Model file for the job. Use its own axes, mm. Give positions to 0.01 mm unless a question says otherwise; leave off trailing zeros. Loops run counter-clockwise (first coordinate to the right, second up) from the corner with the lowest first, then second, coordinate; pieces in that order, holes last. Notation, with made-up numbers: M -15.5,52 L -9.5,52 A31 ccw -9.5,77 Z; hole C 63,83 d5. An arc over 180 degrees is marked long. Answer in a Markdown table with one row per item.
```python
from build123d import *

# Parameters (mm, degrees)
F2_R = 10
F3_R = 2


with BuildPart() as f1:
    # F0 (on Front) → F1 (revolve)
    with BuildSketch(Plane.XZ):
        with BuildLine():
            Line((0, 70), (0, 0))
            Line((0, 0), (25.5, 0))
            Line((25.5, 0), (25.5, 12))
            Line((25.5, 12), (23.161351406, 9.536806494))
            Line((23.161351406, 9.536806494), (12.4268941581, 9.536806494))
            Line((12.4268941581, 9.536806494), (8.2896918707, 17.4999870426))
            Line((8.2896918707, 17.4999870426), (17.8353563403, 54.2824750416))
            add(Edge.make_bspline(
                [(17.8353563403, 54.2824750416), (18.8817362992, 57.6831345085), (19.5978634285, 63.6834766541), (9.8956074759, 68.9451214738), (3.3796710427, 69.9306730781), (0, 70)],
                knots=[0, 0, 0, 0, 0.3192028664, 0.6536802419, 1, 1, 1, 1], degree=3))
        make_face()
    revolve(axis=Axis((0, 0, 35), (0, 0, -1)))

    # F2
    f2_edges = [f1.edges().sort_by_distance(p)[0] for p in [
        (-12.426894, 0, 9.536806),
    ]]
    fillet(f2_edges, radius=F2_R)

    # F3
    f3_edges = [f1.edges().sort_by_distance(p)[0] for p in [
        (-23.161351, 0, 9.536806),
    ]]
    fillet(f3_edges, radius=F3_R)


solid = f1.part
```
(1) Mould opens along Y. For faces 1 (the cylindrical face through (-5.5, 24.9, 6.1)), 2 (the flat face through (0, 0, 0)), 3 (the flat face through (-8, -17, 9.537)) say: pulls with the +Y half, pulls with the -Y half, needs draft (parallel to the pull), parting line crosses it, or undercut.
Established:
| item | result |
|---|---|
| face 1 | parting line crosses it |
| face 2 | needs draft |
| face 3 | undercut |
(2) Saw through at A-A, the plane z = 47. Give the cut face in (x, y), and give its area (3 significant figures).
Established:
| item | result |
|---|---|
| outline | C 0,0 d31.89 |
| area | 799 mm2 |
(3) Saw through at B-B, the plane z = 33. Give the cut face in (x, y).
Established:
| item | result |
|---|---|
| outline | C 0,0 d24.62 |
(4) Wall check: L1, parallel to Z at x = -20, y = -11; L2, parallel to Y at x = -3.5, z = 20; L3, parallel to Z at x = 22.5, y = 11.5. Give the ranges that are in metal, low to high.
Established:
| item | result |
|---|---|
| L1 | z = 0 to 9.61 |
| L2 | y = -8.22 to 8.22 |
| L3 | z = 0 to 11.76 |
(5) Flat gauge pins, fed straight in: P1, Ø8, axis at x = -1.5, z = 9, coming from the +Y side; P2, Ø8, axis at y = -15, z = 46.5, coming from the -X side; P3, Ø8, axis at x = 4, z = 11, coming from the -Y side. Where does each tip first touch, or does it go through?
Established:
| item | result |
|---|---|
| P1 | stops at y = 25.5 |
| P2 | stops at x = -11.62 |
| P3 | stops at y = -25.5 |
